```python
from build123d import *

# Parameters (mm, degrees)
SKETCH1_R                        = 15.875
BOSS_EXTRUDE1_DEPTH              = 23.4696
CUT_EXTRUDE1_START               = -20.32
SKETCH2_R                        = 15.875
SKETCH2_R_2                      = 7.9375
CUT_EXTRUDE1_DEPTH               = 20.32
M6X1_0_TAPPED_HOLE1_D            = 5
F_36_0_1065_DIAMETER_HOLE2_D     = 2.7051
F_36_0_1065_DIAMETER_HOLE2_DEPTH = 6.35
F_36_0_1065_DIAMETER_HOLE2_TIP   = 0.81269403
CUT_EXTRUDE2_DEPTH               = 31.280912305


with BuildPart() as part:
    # Sketch1 → Boss-Extrude1 (new body)
    with BuildSketch(Plane.XY):
        Circle(SKETCH1_R)
    extrude(amount=BOSS_EXTRUDE1_DEPTH)

    # Sketch2 → Cut-Extrude1 (cut)
    with BuildSketch(Plane.XY.offset(23.4696).offset(CUT_EXTRUDE1_START)):
        Circle(SKETCH2_R)
        Circle(SKETCH2_R_2, mode=Mode.SUBTRACT)
    extrude(amount=CUT_EXTRUDE1_DEPTH, mode=Mode.SUBTRACT)

    # M6x1.0 Tapped Hole1 (through all)
    with Locations(Plane.XY.offset(23.4696)):
        with Locations((0, 0)):
            Hole(M6X1_0_TAPPED_HOLE1_D / 2)

    # #36 (0.1065) Diameter Hole2
    with Locations(Plane.XY.offset(3.1496)):
        with Locations((11.90625, 0), (-11.90625, 0)):
            Hole(F_36_0_1065_DIAMETER_HOLE2_D / 2, depth=F_36_0_1065_DIAMETER_HOLE2_DEPTH)
            with Locations((0, 0, -(F_36_0_1065_DIAMETER_HOLE2_DEPTH + F_36_0_1065_DIAMETER_HOLE2_TIP / 2))):  # 118° drill point
                Cone(0, F_36_0_1065_DIAMETER_HOLE2_D / 2, F_36_0_1065_DIAMETER_HOLE2_TIP, mode=Mode.SUBTRACT)

    # Sketch8 → Cut-Extrude2 (cut, through all)
    with BuildSketch(Plane.XY.offset(3.1496)):
        with BuildLine():
            Line((0, 7.9375), (-13.748153285, 7.9375))
            ThreePointArc((-13.748153285, 7.9375), (0, 15.875), (13.748153285, 7.9375))
            Line((13.748153285, 7.9375), (0, 7.9375))
        make_face()
        with BuildLine():
            Line((-13.748153285, -7.9375), (13.748153285, -7.9375))
            ThreePointArc((13.748153285, -7.9375), (0, -15.875), (-13.748153285, -7.9375))
        make_face()
    extrude(amount=-CUT_EXTRUDE2_DEPTH, mode=Mode.SUBTRACT)


solid = part.part
```
Could you check a few things on this model? Use its own coordinates, in mm. Coordinates: 2 decimals unless noted, no trailing zeros. Write each loop counter-clockwise with the first axis right and the second up, starting at its lowest first coordinate (ties: lowest second). Pieces come first, ordered by that corner, then holes. Notation, with made-up numbers: (87.5, 35) -> (116.5, 35) arc R10 cw to (116.5, 41) -> close; hole circle Ø8 at (-16, 62.5). An arc over 180 degrees is marked (long way). Write item = value, one per line. Start each with the question number.
(1) I want a section at D-D (z = 20.5). Please give me the cut outline in (x, y) (1 decimal), plus the area to 3 significant figures.
(2) Will these pins go through, and if not, where does the flat tip stop? pin 1 (12 mm diameter, centred on x = -8, z = 10.5, fed in from -Y); pin 2 (1 mm diameter, centred on y = 2.5, z = 11.5, fed in from +X); pin 3 (3 mm diameter, centred on y = 0, z = 14.5, fed in from +X).
(3) I want a section at C-C (y = -2). Please give me the cut outline in (x, z), plus the area to 3 significant figures.
(4) I need wall thicknesses on line 1 (X direction, y = -1, z = 2.5); line 2 (Y direction, x = 0, z = 5); line 3 (Z direction, x = 11, y = 1.75). Which ranges of each line are inside material? Lowest first, please. Write a range as [from, to].
(5) I want a section at B-B (x = 12). Please give me the cut outline in (y, z).
(6) I want a section at A-A (y = 0). Please give me the cut outline in (x, z) (1 decimal), plus the area to 3 significant figures.
(7) We'd pull the mould along X, two halves only. Please class faces 1 (the face through (-1.72, -7.75, 13.17)), 2 (the face through (-10.555, 0.059, 1.553)), 3 (the face through (13.257, 0.059, 1.553)), 4 (the face through (10, 0, 3.15)): released by +X, released by -X, zero draft, split by the parting line, or undercut.
Result set:
q1.outline = circle Ø15.9 at (0, 0); hole circle Ø5 at (0, 0)
q1.area = 178 mm2
q2.pin_1 = -7.68
q2.pin_2 = 7.68
q2.pin_3 = 7.94
q3.outline = (-15.75, 0) -> (-1.5, 0) -> (-1.5, 23.47) -> (-7.68, 23.47) -> (-7.68, 3.15) -> (-15.75, 3.15) -> close; (1.5, 0) -> (15.75, 0) -> (15.75, 3.15) -> (7.68, 3.15) -> (7.68, 23.47) -> (1.5, 23.47) -> close
q3.area = 341 mm2
q4.line_1 = [-15.84, -12.82], [-11, -2.29], [2.29, 11], [12.82, 15.84]
q4.line_2 = [-7.94, -2.5], [2.5, 7.94]
q4.line_3 = [0, 3.15]
q5.outline = (-7.94, 0) -> (-1.35, 0) -> (-1.35, 3.15) -> (-7.94, 3.15) -> close; (1.35, 0) -> (7.94, 0) -> (7.94, 3.15) -> (1.35, 3.15) -> close
q6.outline = (-15.9, 0) -> (-13.3, 0) -> (-13.3, 3.1) -> (-15.9, 3.1) -> close; (-10.6, 0) -> (-2.5, 0) -> (-2.5, 23.5) -> (-7.9, 23.5) -> (-7.9, 3.1) -> (-10.6, 3.1) -> close; (2.5, 0) -> (10.6, 0) -> (10.6, 3.1) -> (7.9, 3.1) -> (7.9, 23.5) -> (2.5, 23.5) -> close; (13.3, 0) -> (15.9, 0) -> (15.9, 3.1) -> (13.3, 3.1) -> close
q6.area = 288 mm2
q7.face_1 = split by the parting line
q7.face_2 = undercut
q7.face_3 = undercut
q7.face_4 = zero draft
